Autodesk Inventor part; units mm, degrees
ref_plane "YZ Plane" through (0, 0, 0) normal (1, 0, 0) x (0, 1, 0)
ref_plane "XZ Plane" through (0, 0, 0) normal (0, 1, 0) x (-1, 0, 0)
ref_plane "XY Plane" through (0, 0, 0) normal (0, 0, 1) x (1, 0, 0)
sketch "草圖1" plane through (0, 0, 0) normal (0, 0, 1) x (1, 0, 0)
  line L0 (0, 0) -> (-43, 0)
  line L1 (0, 0) -> (0, 6.7073)
  line L2 (0, 6.7073) -> (-1.691, 13.5)
  line L3 (-1.691, 13.5) -> (-36.2631, 13.5)
  arc A0 (-41.5549, 15.0149) -> (-36.2631, 13.5) centre (-36.2631, 23.5) ccw
  arc A1 (-41.5549, 15.0149) -> (-46.6885, 3.2242) centre (-44.9946, 9.4996) ccw
  arc A2 (-44.9289, 1.4714) -> (-46.6885, 3.2242) centre (-47.34, 0.8106) ccw
  arc A3 (-44.9289, 1.4714) -> (-43, 0) centre (-43, 2) ccw
  circle A4 centre (-44.9946, 9.4996) radius 4
  dimension "d0" = 43
  dimension "d1" = 13.5
  dimension "d2" = 10
  dimension "d3" = 2
  dimension "d6" = 2.5
  dimension "d7" = 6.5
  dimension "d8" = 4.899
  dimension "d9" = 2.426
  dimension "d10" = 7
  dimension "d11" = 6.7073
  dimension "d12" = 8
extrude "擠出1" add sketch "草圖1" along normal blind 20
sketch "草圖2" plane through (-36.2631, 13.5, 0) normal (0, 1, 0) x (1, 0, 0)
  line L0 (36.2631, 0) -> (36.2631, -20) construction
  line L1 (34.572, -20) -> (0, -20)
  line L2 (34.572, 0) -> (34.572, -20)
  arc A0 (31.5631, -16) -> (33.5631, -18) centre (33.5631, -16) ccw
  line L3 (31.5631, -16) -> (31.5631, -4)
  arc A1 (33.5631, -2) -> (31.5631, -4) centre (33.5631, -4) ccw
  line L4 (33.5631, -18) -> (4.5631, -18)
  line L5 (33.5631, -2) -> (4.5631, -2)
  arc A2 (4.5631, -18) -> (7.0631, -15.5) centre (4.5631, -15.5) ccw
  line L6 (7.0631, -15.5) -> (7.0631, -4.5)
  arc A3 (7.0631, -4.5) -> (4.5631, -2) centre (4.5631, -4.5) ccw
  circle A4 centre (27.2631, -14.4) radius 1.6
  line L7 (27.2631, -14.4) -> (27.2631, -5.6) construction
  circle A5 centre (27.2631, -5.6) radius 1.6
  line L8 (27.2631, -14.4) -> (15.9631, -14.4) construction
  line L9 (15.9631, -14.4) -> (15.9631, -5.6) construction
  circle A6 centre (15.9631, -14.4) radius 1.6
  circle A7 centre (15.9631, -5.6) radius 1.6
  circle A8 centre (10.8631, -10) radius 1.6
  line L10 (33.5631, -18) -> (36.2631, -18)
  line L11 (36.2631, 0) -> (36.2631, -20)
  line L12 (33.5631, -2) -> (36.2631, -2)
  line L13 (36.2631, -18) -> (36.2631, -2)
  line L14 (-15.2315, 0) -> (-15.2315, -20)
  line L15 (4.5631, -18) -> (-15.2315, -18)
  line L16 (4.5631, -2) -> (-15.2315, -2)
  line L17 (-15.2315, -18) -> (-15.2315, -2)
  dimension "d22" = 2
  dimension "d24" = 2
  dimension "d25" = 2
  dimension "d26" = 4.7
  dimension "d27" = 16
  dimension "d28" = 29
  dimension "d29" = 2.5
  dimension "d30" = 2.5
  dimension "d31" = 3.2
  dimension "d32" = 4.3
  dimension "d33" = 3.6
  dimension "d34" = 8.8
  dimension "d35" = 11.3
  dimension "d36" = 8.8
  dimension "d38" = 23.709
  dimension "d39" = 10
extrude "擠出2" cut sketch "草圖2" against normal blind 11.5 contours A1 L3 A0 L4 A2 L6 A3 L5 | A4 | A5 | A6 | A7 | A8
extrude "擠出3" cut sketch "草圖2" against normal through all contours A4 | A5 | A6 | A7 | A8
extrude "擠出4" cut sketch "草圖2" along normal through all both and the other way through all contours L12 L11 L10 L2 | L2 L10 A0 L3 A1 L12 | A3 L6 A2 L15 L14 L16
sketch "草圖3" plane through (0, 0, 0) normal (0, 0, -1) x (-1, 0, 0)
  line L0 (0, 6.7073) -> (0, 0)
  line L1 (0, 6.7073) -> (7.7777, 37.9495)
  line L2 (0, 6.7073) -> (1.691, 13.5)
  arc A0 (19.6, 36.5) -> (7.7777, 37.9495) centre (13.6, 36.5) ccw
  line L3 (19.6, 36.5) -> (19.6, 13.5)
  line L4 (19.6, 13.5) -> (0, 6.7073)
  line L5 (43, 0) -> (0, 0)
  circle A1 centre (13.6, 36.5) radius 1.65
  dimension "d46" = 36.5
  dimension "d47" = 6
  dimension "d48" = 23
  dimension "d49" = 3.3
extrude "擠出5" add sketch "草圖3" against normal blind 2
fillet "圓角1" radius 1 2 edges at (0, 0, 19) (0, 0, 1)
fillet "圓角1" radius 5 2 edges at (0, 6.7073, 19) (0, 6.7073, 1)
fillet "圓角1" radius 2 1 edges at (-1.691, 13.5, 19)
properties part number "front joint"
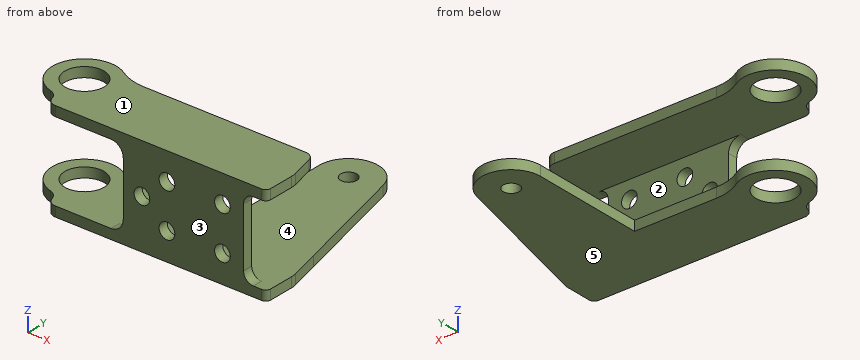
Verification items for the finished model (mm, model axes). Face numbers are marked on the shaded views. A direction names the side the tool comes from. Round coordinates to 2 decimals unless told otherwise and drop trailing zeros. Order: outer loops, then holes, each group sorted by start corner. A loop starts at its lowest first (then second) coordinate and runs counter-clockwise, first axis right, second up.
1. Release check for a two-part mould opening along Z. For the marked faces 3, 4 and 5 record: +Z half, -Z half, draft (parallel to the pull), parting line (faces both ways), or undercut.
Final values:
face 3: draft
face 4: undercut
face 5: -Z half
2. Thickness scan on L1, parallel to Z at x = -49, y = 4.5; L2, parallel to X at y = 0.75, z = 14.4; L3, parallel to Y at x = -13.6, z = 0.75. Record the ranges inside material, lowest first.
Final values:
L1: z = 0 to 2, 18 to 20
L2: x = -29.2 to -21.9, -18.7 to -10.6, -7.4 to -4.7
L3: y = 0 to 34.85, 38.15 to 42.5
3. Section check C-C on y = 8.5. Record the cut outline in (x, z).
Final values:
outline: (-51.42, 0) - (-48.87, 0) - (-48.87, 2) - (-51.42, 2) - close; (-51.42, 18) - (-48.87, 18) - (-48.87, 20) - (-51.42, 20) - close; (-41.12, 0) - (-0.45, 0) - (-0.45, 2) - (-41.12, 2) - close; (-41.12, 18) - (-0.45, 18) - (-0.45, 20) - (-41.12, 20) - close
4. Section check A-A on z = 14.4. Record the cut outline in (x, y).
Final values:
outline: (-29.2, 0) - (-21.9, 0) - (-21.9, 2) - (-29.2, 2) - close; (-18.7, 0) - (-10.6, 0) - (-10.6, 2) - (-18.7, 2) - close; (-7.4, 0) - (-4.7, 0) - (-4.7, 2) - (-7.4, 2) - close
5. Go/stop test with flat-tipped pins: P1, Ø4, axis at x = -26, z = 13, coming from the +Y side; P2, Ø1.9, axis at x = -20.3, z = 14.4, coming from the +Y side; P3, Ø1.5, axis at x = -11, z = 5, coming from the -Y side; P4, Ø2, axis at x = -31, z = 1, coming from the +Y side. Record where each tip stops, or that it passes through.
Final values:
P1: stops at y = 2
P2: passes through
P3: stops at y = 0
P4: stops at y = 13.5
6. Section check D-D on z = 10. Record the cut outline in (x, y).
Final values:
outline: (-29.2, 0) - (-27, 0) - (-27, 2) - (-29.2, 2) - close; (-23.8, 0) - (-4.7, 0) - (-4.7, 2) - (-23.8, 2) - close
7. Section check B-B on x = -20.3. Record the cut outline in (y, z).
Final values:
outline: (0, 0) - (13.5, 0) - (13.5, 2) - (2, 2) - (2, 4) - (0, 4) - close; (0, 7.2) - (2, 7.2) - (2, 12.8) - (0, 12.8) - close; (0, 16) - (2, 16) - (2, 18) - (13.5, 18) - (13.5, 20) - (0, 20) - close
8. Access from +Z, -Z, +X, -X, +Y, -Y to the whole of each face (thin tool, end or side, straight path). Record for the marked faces 1 and 2.
Final values:
face 1: +Z, +X, -X, +Y, -Y
face 2: +X, -X, +Y
